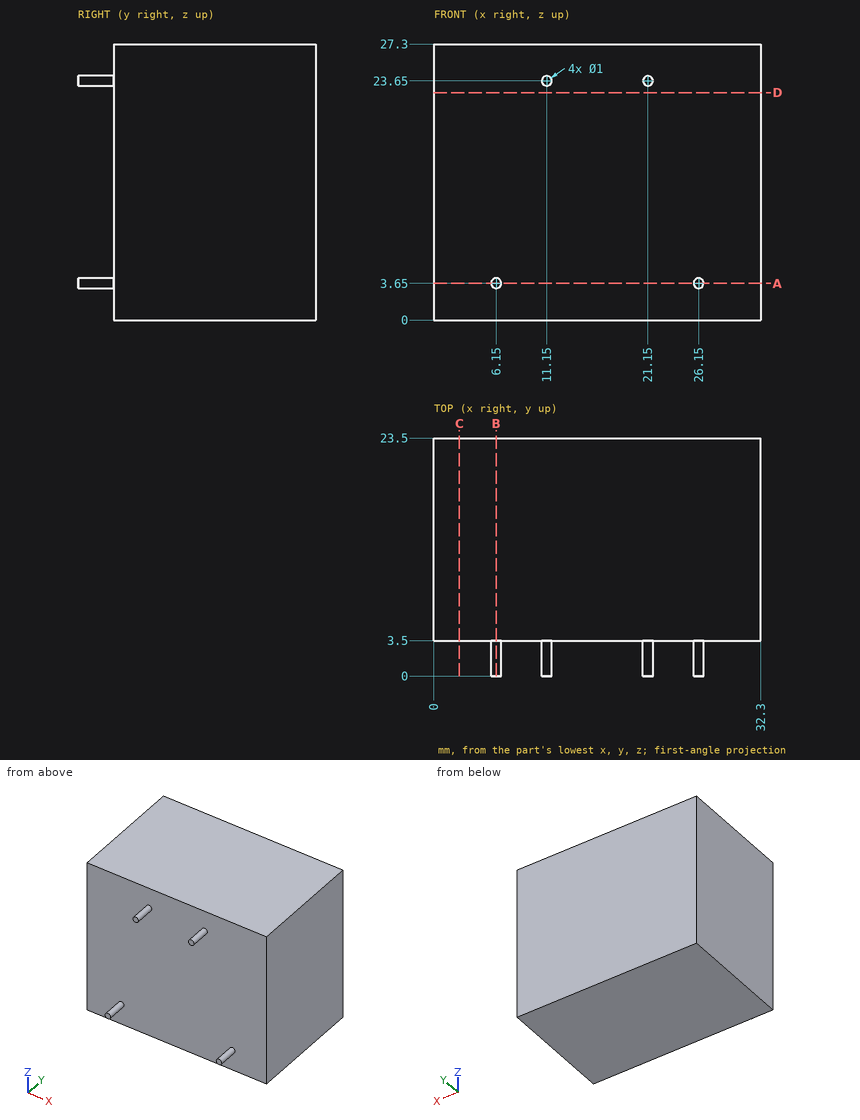
Source: three-view drawing plus pictorial views. Frame: mm from the lowest corner of the part. Round coordinates to 2 decimals unless told otherwise and drop trailing zeros. Loops run counter-clockwise (first coordinate to the right, second up) from the corner with the lowest first, then second, coordinate; pieces in that order, holes last. Notation, with made-up numbers: M 60.25,12 L 72.25,12 A24 ccw 72.25,28 Z; hole C -26.5,12.5 d5. An arc over 180 degrees is marked long. Answer as CSV lines item,"result". Start each with the question number.
(1) Section D-D, the plane z = 22.5. Output: boundary loops of the cut face in (x, y), plus the area to 3 significant figures.
(2) Section B-B, the plane x = 6.15. Output: boundary loops of the cut face in (y, z).
(3) First-contact query: pin 1 (12 mm diameter, centred on x = 12, z = 15.5, fed in from -Y). Flat tip, straight axial feed; report the tip coordinate or a pass-through.
(4) Section A-A, the plane z = 3.65. Output: boundary loops of the cut face in (x, y).
(5) Line query: line 1 (Y direction, x = 13, z = 15.75). Output: solid intervals per line, ascending. Write a range as [from, to].
(6) Section C-C, the plane x = 2.5. Output: boundary loops of the cut face in (y, z).
Values found:
1,outline,"M 0,3.5 L 32.3,3.5 L 32.3,23.5 L 0,23.5 Z"
1,area,"646 mm²"
2,outline,"M 0,3.15 L 3.5,3.15 L 3.5,0 L 23.5,0 L 23.5,27.3 L 3.5,27.3 L 3.5,4.15 L 0,4.15 Z"
3,pin 1,"stops at y = 3.5"
4,outline,"M 0,3.5 L 5.65,3.5 L 5.65,0 L 6.65,0 L 6.65,3.5 L 25.65,3.5 L 25.65,0 L 26.65,0 L 26.65,3.5 L 32.3,3.5 L 32.3,23.5 L 0,23.5 Z"
5,line 1,"y = [3.5, 23.5]"
6,outline,"M 3.5,0 L 23.5,0 L 23.5,27.3 L 3.5,27.3 Z"
